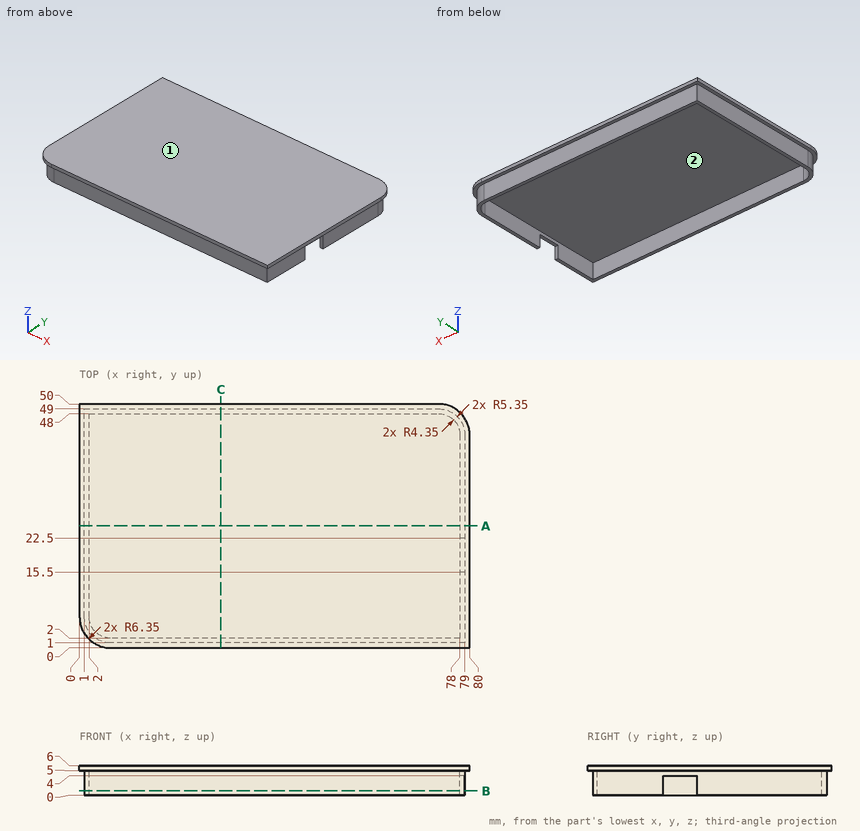
Study the drawing (mm; zero at the part's minimum x, y, z) and answer. Give positions to 0.01 mm unless a question says otherwise; leave off trailing zeros. Loops run counter-clockwise (first coordinate to the right, second up) from the corner with the lowest first, then second, coordinate; pieces in that order, holes last. Notation, with made-up numbers: (36, 84) - (50, 84) arc R25 ccw to (50, 103) - close; hole circle Ø10 at (-9.75, 23). An arc over 180 degrees is marked (long way). Use CSV: the item, a comma, the result in double quotes. Start each with the question number.
(1) Find section B-B, the plane z = 0.85. Determine the outline of the cut face in (x, y).
(2) Find the intervals of material crossed by L1, parallel to Y at x = 57.5, z = 2; L2, parallel to X at y = 36, z = 1.7; L3, parallel to Z at x = 47, y = 18, in increasing order.
(3) Find section C-C, the plane x = 29. Determine the outline of the cut face in (y, z).
(4) Determine the mould class of the marked faces 1 and 2 for opening direction X: released by +X, released by -X, zero draft, split by the parting line, or undercut.
(5) Each of these flat-tipped pins is pushed along its axis until it touches: pin 1 (1.5 mm diameter, centred on x = 60, z = 3.5, fed in from +Y); pin 2 (1.1 mm diameter, centred on x = 78.5, y = 18, fed in from -Z); pin 3 (1.5 mm diameter, centred on y = 16.5, z = 3.5, fed in from +X). Where does it stop, or does it pass through?
(6) Find section A-A, the plane y = 25. Determine the outline of the cut face in (x, z), plus the area to 3 significant figures.
Results found:
1,outline,"(1, 6.35) arc R5.35 ccw to (6.35, 1) - (79, 1) - (79, 15.5) - (78, 15.5) - (78, 2) - (6.35, 2) arc R4.35 cw to (2, 6.35) - (2, 48) - (73.65, 48) arc R4.35 cw to (78, 43.65) - (78, 22.5) - (79, 22.5) - (79, 43.65) arc R5.35 ccw to (73.65, 49) - (1, 49) - close"
2,L1,"1 to 2, 48 to 49"
2,L2,"1 to 2, 78 to 79"
2,L3,"5 to 6"
3,outline,"(0, 5) - (1, 5) - (1, 0) - (2, 0) - (2, 5) - (48, 5) - (48, 0) - (49, 0) - (49, 5) - (50, 5) - (50, 6) - (0, 6) - close"
4,face 1,"zero draft"
4,face 2,"undercut"
5,pin 1,"y = 49"
5,pin 2,"z = 4"
5,pin 3,"x = 79"
6,outline,"(0, 5) - (1, 5) - (1, 0) - (2, 0) - (2, 5) - (78, 5) - (78, 0) - (79, 0) - (79, 5) - (80, 5) - (80, 6) - (0, 6) - close"
6,area,"90.0 mm^2"
